Autodesk Inventor part; units mm, degrees
ref_plane "YZ Plane" through (0, 0, 0) normal (1, 0, 0) x (0, 1, 0)
ref_plane "XZ Plane" through (0, 0, 0) normal (0, 1, 0) x (-1, 0, 0)
ref_plane "XY Plane" through (0, 0, 0) normal (0, 0, 1) x (1, 0, 0)
sketch "Sketch1" plane through (0, 0, 0) normal (0, 0, 1) x (1, 0, 0)
  line L0 (0, 0) -> (9.525, 0)
  line L1 (9.525, 0) -> (9.525, 25.4)
  line L2 (9.525, 25.4) -> (0, 25.4)
  line L3 (0, 25.4) -> (0, 0)
  dimension "d0" = 9.525
  dimension "d1" = 25.4
extrude "Extrusion1" add sketch "Sketch1" along normal blind 60.325
sketch "Sketch2" plane through (0, 25.4, 0) normal (0, 1, 0) x (1, 0, 0)
  line L0 (0, 0) -> (0, -60.325) construction
  line L1 (9.525, -60.325) -> (0, -60.325) construction
  line L2 (0, -30.1625) -> (9.525, -30.1625) construction
  point P0 (4.7625, -53.975)
  point P1 (4.7625, -6.35)
  dimension "d4" = 4.7625
  dimension "d5" = 6.35
hole "Hole1" at (4.7625, 25.4, 53.975) at (4.7625, 25.4, 6.35) direction (0, -1, 0) diameter 3.302 end through all
properties part number "ImagineFrameSides" material "SAN Plastic"
For this review, take the finished solid that the model builds, in its own axes (mm). Round coordinates to 2 decimals unless told otherwise and drop trailing zeros. Write each loop counter-clockwise with the first axis right and the second up, starting at its lowest first coordinate (ties: lowest second). Pieces come first, ordered by that corner, then holes. Notation, with made-up numbers: (-34, 6.5) - (-9, 6.5) arc R22 cw to (-9, 34.5) - close; hole circle Ø1 at (67, -5.75). An arc over 180 degrees is marked (long way). Use a Markdown table: item, result.
Q1. We need section B-B (y = 13.5). State how many separate pieces and enclosed holes the cut face has, plus the area to 3 significant figures.
Derived:
| item | result |
|---|---|
| separate pieces | 1 |
| enclosed holes | 2 |
| area | 557 mm2 |
Q2. Wall thickness on line 1 along X through (y, z) = (9.75, 6.35) (1 decimal); line 2 along Z through (x, y) = (3.5, 16) (3 decimals); line 3 along Z through (x, y) = (5, 10.75) (3 decimals): over which ranges is each line inside the solid? List them lowest first.
Derived:
| item | result |
|---|---|
| line 1 | x = 0 to 3.1, 6.4 to 9.5 |
| line 2 | z = 0 to 5.286, 7.414 to 52.911, 55.039 to 60.325 |
| line 3 | z = 0 to 4.716, 7.984 to 52.341, 55.609 to 60.325 |
Q3. Clearance check with a flat-ended pin moving along its axis: pin 1 (5 mm diameter, centred on x = 1, z = 28, fed in from -Y). State where the tip first meets the part, or that it passes through.
Derived:
| item | result |
|---|---|
| pin 1 | stops at y = 0 |
Q4. We need section A-A (z = 6.35). Give the boundary of the cut face in (x, y) (1 decimal), plus the area to 3 significant figures.
Derived:
| item | result |
|---|---|
| outline | (0, 0) - (3.1, 0) - (3.1, 25.4) - (0, 25.4) - close; (6.4, 0) - (9.5, 0) - (9.5, 25.4) - (6.4, 25.4) - close |
| area | 158 mm2 |
Q5. The part is to be moulded in two halves that separate along X. For faces 1 (the cylindrical face through (3.37, 12.52, 7.24)), 2 (the flat face through (0, 13, 30)), 3 (the flat face through (5, 0, 30)), say which applies: pulls with the +X half, pulls with the -X half, needs draft (parallel to the pull), parting line crosses it, or undercut.
Derived:
| item | result |
|---|---|
| face 1 | undercut |
| face 2 | pulls with the -X half |
| face 3 | needs draft |
